Input: part model. Units: mm. Frame: model coordinates. Give positions to 0.01 mm unless a question says otherwise; leave off trailing zeros. Loops run counter-clockwise (first coordinate to the right, second up) from the corner with the lowest first, then second, coordinate; pieces in that order, holes last.
from build123d import *

# Parameters (mm, degrees)
SKETCH1_W           = 200
SKETCH1_H           = 100
BOSS_EXTRUDE1_DEPTH = 3.36
SKETCH9_W           = 3.44
SKETCH9_H           = 50
BOSS_EXTRUDE5_DEPTH = 3.36
SKETCH10_W          = 100
SKETCH10_H          = 3.28
CUT_EXTRUDE1_DEPTH  = 3.36


with BuildPart() as part:
    # Sketch1 → Boss-Extrude1 (new body)
    with BuildSketch(Plane.XY):
        Rectangle(SKETCH1_W, SKETCH1_H)
    extrude(amount=BOSS_EXTRUDE1_DEPTH)

    # Sketch9 → Boss-Extrude5 (add)
    with BuildSketch(Plane(origin=(0, 0, 0), x_dir=(-1, 0, 0), z_dir=(0, 0, -1))):
        with Locations((101.72, 0)):
            Rectangle(SKETCH9_W, SKETCH9_H)
    boss_extrude5 = extrude(amount=-BOSS_EXTRUDE5_DEPTH)

    # Mirror5: Boss-Extrude5 across plane
    add(boss_extrude5.mirror(Plane(origin=(0, 0, 0), x_dir=(0, 0, 1), z_dir=(1, 0, 0))))

    # Sketch10 → Cut-Extrude1 (cut)
    with BuildSketch(Plane.XY.offset(3.36)):
        with Locations((0, 48.36)):
            Rectangle(SKETCH10_W, SKETCH10_H)
    cut_extrude1 = extrude(amount=-CUT_EXTRUDE1_DEPTH, mode=Mode.SUBTRACT)

    # Mirror6: Cut-Extrude1 across plane
    add(cut_extrude1.mirror(Plane.ZX), mode=Mode.SUBTRACT)


solid = part.part
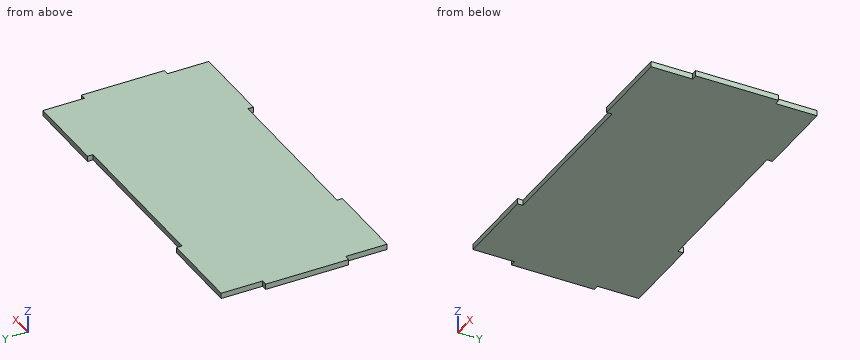
(1) Cut plane C-C (x = 14). Return the cut outline in (y, z), and give its area (3 significant figures).
Values follow:
outline: (-46.72, 0) - (46.72, 0) - (46.72, 3.36) - (-46.72, 3.36) - close
area: 314 mm2
(2) Cut plane B-B (y = -37.5). Return the cut outline in (x, z).
Values follow:
outline: (-100, 0) - (100, 0) - (100, 3.36) - (-100, 3.36) - close
(3) Ray query, probe 1 along X at (y, z) = (38.5, 2.05); probe 2 along Y at (x, z) = (48, 1.6). Return the intervals inside material, ascending.
Values follow:
probe 1: x = -100 to 100
probe 2: y = -46.72 to 46.72
(4) Pin query (flat end, axial travel): pin 1 Ø1 at (y, z) = (-49, 1.5) entering from -X; pin 2 Ø1.7 at (x, z) = (101.5, 1) entering from -Y; pin 3 Ø1 at (y, z) = (35, 2) entering from +X; pin 4 Ø1 at (x, y) = (-66, 28.5) entering from -Z. Return the tip coordinate at first contact, or that it passes through.
Values follow:
pin 1: stops at x = -100
pin 2: stops at y = -25
pin 3: stops at x = 100
pin 4: stops at z = 0
(5) Cut plane A-A (z = 1.25). Return the cut outline in (x, y).
Values follow:
outline: (-103.44, -25) - (-100, -25) - (-100, -50) - (-50, -50) - (-50, -46.72) - (50, -46.72) - (50, -50) - (100, -50) - (100, -25) - (103.44, -25) - (103.44, 25) - (100, 25) - (100, 50) - (50, 50) - (50, 46.72) - (-50, 46.72) - (-50, 50) - (-100, 50) - (-100, 25) - (-103.44, 25) - close
